Part print with two shaded views. Sizes in mm from the minimum x, y, z corner. A direction names the side the tool comes from. Round coordinates to 2 decimals unless told otherwise and drop trailing zeros. Order: outer loops, then holes, each group sorted by start corner. A loop starts at its lowest first (then second) coordinate and runs counter-clockwise, first axis right, second up. Notation, with made-up numbers: (84, 80) - (107, 80) arc R20 cw to (107, 104) - close; hole circle Ø10 at (-18, -11). An arc over 180 degrees is marked (long way). Use one line per item in the form item = value.
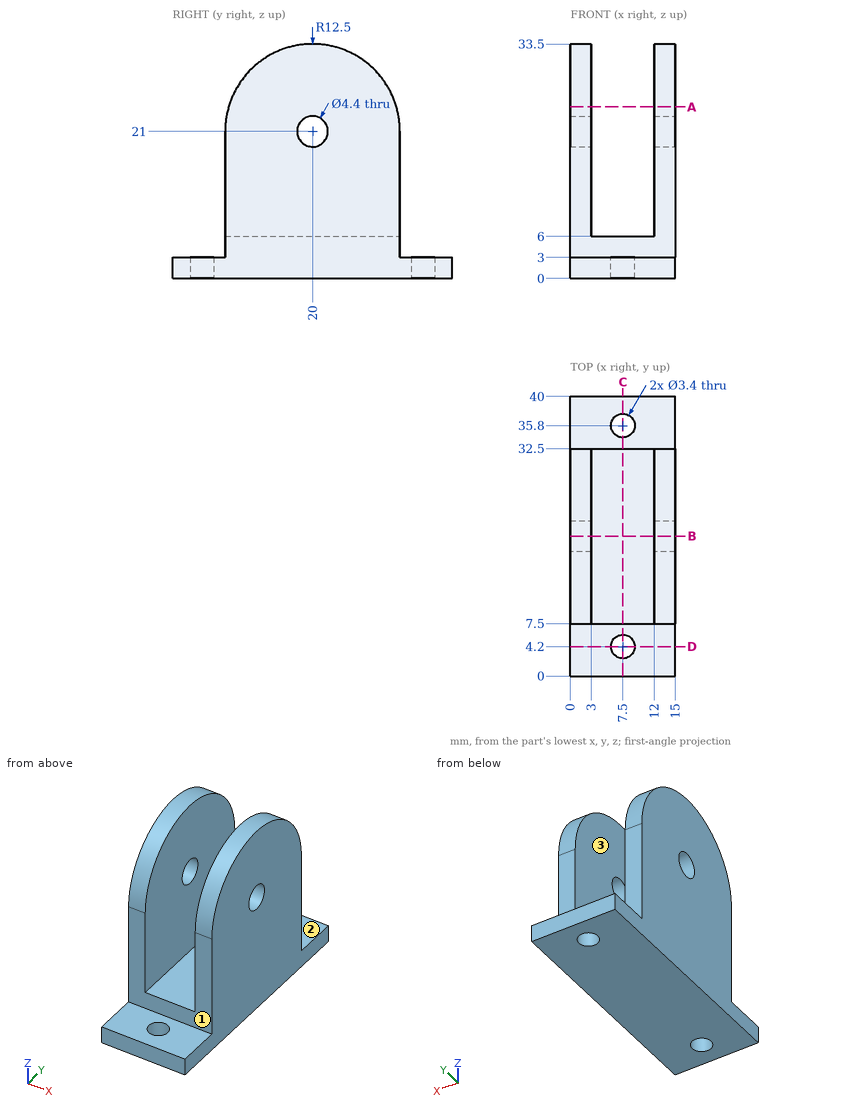
(1) Slice it at C-C on x = 7.5. Give the cut face in (y, z).
Report:
outline = (0, 0) - (2.5, 0) - (2.5, 3) - (0, 3) - close; (5.9, 0) - (34.1, 0) - (34.1, 3) - (32.5, 3) - (32.5, 6) - (7.5, 6) - (7.5, 3) - (5.9, 3) - close; (37.5, 0) - (40, 0) - (40, 3) - (37.5, 3) - close
(2) Tool access for the marked faces 1, 2 and 3: list every direction of +Z, -Z, +X, -X, +Y, -Y with a clear straight run to the whole face (end or side of a thin tool).
Report:
face_1 = +Z, +X, -X, -Y
face_2 = +Z, +X, -X, +Y
face_3 = +Z, +Y, -Y
(3) Probe probe 1 along Y at (x, z) = (7.5, 1.85); probe 2 along Z at (x, y) = (1.75, 20); probe 3 along Y at (x, z) = (2.15, 21). List the from-to ranges inside material, lowest first. Write a range as [from, to].
Report:
probe_1 = [0, 2.5], [5.9, 34.1], [37.5, 40]
probe_2 = [0, 18.8], [23.2, 33.5]
probe_3 = [7.5, 17.8], [22.2, 32.5]
(4) Slice it at D-D on y = 4.2. Give the cut face in (x, z), then the cut area to 3 significant figures.
Report:
outline = (0, 0) - (5.8, 0) - (5.8, 3) - (0, 3) - close; (9.2, 0) - (15, 0) - (15, 3) - (9.2, 3) - close
area = 34.8 mm2
(5) Pin check, flat tips, straight feed: pin 1 (6 mm diameter, centred on x = 8.5, y = 37, fed in from +Z); pin 2 (4.5 mm diameter, centred on x = 7, y = 14.5, fed in from +Z); pin 3 (1.5 mm diameter, centred on x = 2.5, z = 21.5, fed in from +Y). Stop position of each tip, or through.
Report:
pin_1 = 3
pin_2 = 6
pin_3 = 32.5
(6) Slice it at B-B on y = 20. Give the cut face in (x, z), then the cut area to 3 significant figures.
Report:
outline = (0, 0) - (15, 0) - (15, 18.8) - (12, 18.8) - (12, 6) - (3, 6) - (3, 18.8) - (0, 18.8) - close; (0, 23.2) - (3, 23.2) - (3, 33.5) - (0, 33.5) - close; (12, 23.2) - (15, 23.2) - (15, 33.5) - (12, 33.5) - close
area = 229 mm2
(7) Slice it at A-A on z = 24.5. Give the cut face in (x, y).
Report:
outline = (0, 8) - (3, 8) - (3, 32) - (0, 32) - close; (12, 8) - (15, 8) - (15, 32) - (12, 32) - close
